from build123d import *

# Parameters (mm, degrees)
F0_W          = 23
F0_H          = 17.5
F1_DEPTH      = 10
F2_T          = -1.2
F3_R          = 5.7
F4_DEPTH      = 3
F3_R_2        = 6.7
F5_DEPTH      = 7.5
F6_W          = 6
F6_H          = 2.3
F6_W_2        = 3.5
F6_H_2        = 3.5
F7_DEPTH      = 4
F8_DEPTH      = 3
F10_DEPTH     = 30
F11_T1_DEPTH  = 19
F11_T3_DEPTH  = 23.5
F11_T5_DEPTH  = 13
F11_T7_DEPTH  = 27.8205080757
F11_S11_W     = 2
F11_S11_H     = 2
F11_T12_DEPTH = 2
F11_S17_W     = 2
F11_S17_H     = 2
F11_T18_DEPTH = 2


# Not quite as in the source:
# - a fillet or chamfer that OpenCascade refuses, or shapes differently, is made with other operations: its cross-section is extruded or revolved along the edge and cut away or added


with BuildPart() as f1:
    # F0 (on Front) → F1 (new body)
    with BuildSketch(Plane.XZ):
        Rectangle(F0_W, F0_H)
    extrude(amount=F1_DEPTH)

    # F2
    f2_openings = [f1.faces().sort_by_distance(p)[0] for p in [
        (0, -10, 0),
    ]]
    offset(amount=F2_T, openings=f2_openings)

    # F3 (on face) → F4 (cut)
    with BuildSketch(Plane(origin=(0, 0, 0), x_dir=(-1, 0, 0), z_dir=(0, 1, 0))):
        Circle(F3_R)
    extrude(amount=-F4_DEPTH, mode=Mode.SUBTRACT)

    # F3 (on face) → F5 (join)
    with BuildSketch(Plane(origin=(0, 0, 0), x_dir=(-1, 0, 0), z_dir=(0, 1, 0))):
        Circle(F3_R_2)
        Circle(F3_R, mode=Mode.SUBTRACT)
    extrude(amount=F5_DEPTH)

    # F6 (on face) → F7 (cut)
    with BuildSketch(Plane.XY.offset(8.75)):
        with Locations((1.5, -8.85)):
            Rectangle(F6_W, F6_H)
        with Locations((-5.75, -8.25)):
            Rectangle(F6_W_2, F6_H_2)
    extrude(amount=-F7_DEPTH, mode=Mode.SUBTRACT)

    # F8 (add): a face of the model
    f8_faces = [f1.faces().sort_by_distance(p)[0] for p in [
        (0, -5, -8.75),
    ]]
    extrude(f8_faces, amount=F8_DEPTH)

    # F9 (on face) → F10 (cut)
    with BuildSketch(Plane.YZ.offset(11.5)):
        Polygon((-10, -11.75), (0, -11.75), (-10, -9.0705080757), align=None)
    extrude(amount=-F10_DEPTH, mode=Mode.SUBTRACT)

    # F11: fillet of radius 2 on 7 edges, made by hand

    # F11_s2 → F11_t1 (cut)
    with BuildSketch(Plane.YZ.offset(-9.5)):
        with BuildLine():
            ThreePointArc((0, 6.75), (-0.5857864376, 8.1642135624), (-2, 8.75))
            Line((-2, 8.75), (0, 8.75))
            Line((0, 8.75), (0, 6.75))
        make_face()
    extrude(amount=F11_T1_DEPTH, mode=Mode.SUBTRACT)

    # F11_s4 → F11_t3 (cut)
    with BuildSketch(Plane.XY.offset(-16.75)):
        with BuildLine():
            ThreePointArc((-11.5, -2), (-10.9142135624, -0.5857864376), (-9.5, 0))
            Line((-9.5, 0), (-11.5, 0))
            Line((-11.5, 0), (-11.5, -2))
        make_face()
        with BuildLine():
            ThreePointArc((9.5, 0), (10.9142135624, -0.5857864376), (11.5, -2))
            Line((11.5, -2), (11.5, 0))
            Line((11.5, 0), (9.5, 0))
        make_face()
    extrude(amount=F11_T3_DEPTH, mode=Mode.SUBTRACT)

    # F11_s6 → F11_t5 (cut)
    with BuildSketch(Plane.XZ.offset(2)):
        with BuildLine():
            ThreePointArc((9.5, 8.75), (10.9142135624, 8.1642135624), (11.5, 6.75))
            Line((11.5, 6.75), (11.5, 8.75))
            Line((11.5, 8.75), (9.5, 8.75))
        make_face()
        with BuildLine():
            ThreePointArc((-11.5, 6.75), (-10.9142135624, 8.1642135624), (-9.5, 8.75))
            Line((-9.5, 8.75), (-11.5, 8.75))
            Line((-11.5, 8.75), (-11.5, 6.75))
        make_face()
    extrude(amount=F11_T5_DEPTH, mode=Mode.SUBTRACT)

    # F11_s8 → F11_t7 (cut)
    with BuildSketch(Plane.XY.offset(-14.0705080757)):
        with BuildLine():
            ThreePointArc((-11.5, -8), (-10.9142135624, -9.4142135624), (-9.5, -10))
            Line((-9.5, -10), (-11.5, -10))
            Line((-11.5, -10), (-11.5, -8))
        make_face()
        with BuildLine():
            ThreePointArc((9.5, -10), (10.9142135624, -9.4142135624), (11.5, -8))
            Line((11.5, -8), (11.5, -10))
            Line((11.5, -10), (9.5, -10))
        make_face()
    extrude(amount=F11_T7_DEPTH, mode=Mode.SUBTRACT)


with BuildPart() as f11_tool10:
    # F11_s11 → F11_t12 (new body)
    with BuildSketch(Plane.XZ.offset(2)):
        with Locations((10.5, 7.75)):
            Rectangle(F11_S11_W, F11_S11_H)
    extrude(amount=-F11_T12_DEPTH)

    # F11_s13 → F11_t14 (revolve, cut)
    with BuildSketch(Plane(origin=(9.5, -2, 6.75), x_dir=(-0.7071067812, 0, -0.7071067812), z_dir=(0.7071067812, 0, -0.7071067812))):
        with BuildLine():
            ThreePointArc((0, -2), (2, 0), (0, 2))
            Line((0, 2), (0, -2))
        make_face()
    revolve(axis=Axis((9.5, -2, 6.75), (0, 1, 0)), mode=Mode.SUBTRACT)


with BuildPart() as f1_1:
    add(f1.part)

    # F11_t9: cut F11_tool10
    add(f11_tool10.part, mode=Mode.SUBTRACT)


with BuildPart() as f11_tool16:
    # F11_s17 → F11_t18 (new body)
    with BuildSketch(Plane.YZ.offset(-9.5)):
        with Locations((-1, 7.75)):
            Rectangle(F11_S17_W, F11_S17_H)
    extrude(amount=-F11_T18_DEPTH)

    # F11_s19 → F11_t20 (revolve, cut)
    with BuildSketch(Plane(origin=(-9.5, -2, 6.75), x_dir=(0, -0.7071067812, -0.7071067812), z_dir=(0, 0.7071067812, -0.7071067812))):
        with BuildLine():
            ThreePointArc((0, -2), (2, 0), (0, 2))
            Line((0, 2), (0, -2))
        make_face()
    revolve(axis=Axis((-9.5, -2, 6.75), (-1, 0, 0)), mode=Mode.SUBTRACT)


with BuildPart() as f1_2:
    add(f1_1.part)

    # F11_t15: cut F11_tool16
    add(f11_tool16.part, mode=Mode.SUBTRACT)


solid = f1_2.part
Read the model definition and answer for the solid it produces. Units are mm, in the model's axes. A direction names the side the tool comes from. Give positions to 0.01 mm unless a question says otherwise; leave off trailing zeros. Write each loop counter-clockwise with the first axis right and the second up, starting at its lowest first coordinate (ties: lowest second). Pieces come first, ordered by that corner, then holes. Notation, with made-up numbers: (42, 52) -> (93, 52) arc R22 ccw to (93, 86) -> close; hole circle Ø4 at (18.25, 11). An arc over 180 degrees is marked (long way). Answer as a JSON object with one key per item and string values. Group by question number.
1) Find section C-C (y = 4.25). Write down the section's boundary in (x, z), and give its area (3 significant figures).
2) Find section A-A (x = 0). Write down the section's boundary in (y, z).
3) Each of these flat-tipped pins is pushed along its axis until it touches: P1, Ø5, axis at y = 3, z = -5.5, coming from the +X side; P2, Ø2, axis at x = -9, z = 1.5, coming from the -Y side; P3, Ø6, axis at x = 2, y = 2.5, coming from the +Z side. Where does it stop, or does it pass through?
4) Consider L1, parallel to X at y = -4.25, z = -6.5; L2, parallel to Y at x = -8.75, z = -1.25; L3, parallel to X at y = -8.75, z = -6. Determine where each line is inside the solid, lowest interval first. Write a range as from..to.
5) The mould has two halves that part along X. Classify faces 4 (the flat face through (-7.5, -8, 8)), 5 (the flat face through (0, -10, -8)), 6 (the flat face through (-4, -8, 8)), 7 (the cylindrical face through (-11.15, -9.13, -0.56)): +X half, -X half, draft (parallel to the pull), parting line (faces both ways), or undercut.
6) Find section D-D (z = -6). Write down the section's boundary in (x, y), and give its area (3 significant figures).
7) A tool of negligible diameter and unlimited length cuts with its end or side. For faces 1 (the flat face through (0, -5, 8.75)), 2 (the flat face through (-4.7, -1.2, 3.5)), 3 (the flat face through (-2.2, 0, -6.5)), from which of +Z, -Z, +X, -X, +Y, -Y can it reach the whole face along a straight path? Write none if from no direction.
8) Find section B-B (z = 0). Write down the section's boundary in (x, y).
Values follow:
{
 "1": {"outline": "circle Ø13.4 at (0, 0); hole circle Ø11.4 at (0, 0)", "area": "39.0 mm2"},
 "2": {"outline": "(-10, -9.07) -> (0, -11.75) -> (0, -6.7) -> (7.5, -6.7) -> (7.5, -5.7) -> (-1.2, -5.7) -> (-1.2, -7.55) -> (-10, -7.55) -> close; (-7.7, 7.55) -> (-1.2, 7.55) -> (-1.2, 5.7) -> (7.5, 5.7) -> (7.5, 6.7) -> (0, 6.7) -> (0, 6.75) arc R2 ccw to (-2, 8.75) -> (-7.7, 8.75) -> close"},
 "3": {"P1": "stops at x = 5.99", "P2": "stops at y = -1.2", "P3": "stops at z = 8.07"},
 "4": {"L1": "x = -11.5..-10.3, 10.3..11.5", "L2": "y = -1.2..0", "L3": "x = -11.35..-10.3, 10.3..11.35"},
 "5": {"face 4": "undercut", "face 5": "draft", "face 6": "undercut", "face 7": "-X half"},
 "6": {"outline": "(-11.5, -8) arc R2 ccw to (-10.3, -9.83) -> (-10.3, -1.2) -> (10.3, -1.2) -> (10.3, -9.83) arc R2 ccw to (11.5, -8) -> (11.5, -2) arc R2 ccw to (9.5, 0) -> (2.98, 0) -> (2.98, 7.5) -> (-2.98, 7.5) -> (-2.98, 0) -> (-9.5, 0) arc R2 ccw to (-11.5, -2) -> close", "area": "90.1 mm2"},
 "7": {"face 1": "+Z, +X, -X, +Y, -Y", "face 2": "-Y", "face 3": "+Y"},
 "8": {"outline": "(-11.5, -8) arc R2 ccw to (-10.3, -9.83) -> (-10.3, -1.2) -> (-5.7, -1.2) -> (-5.7, 7.5) -> (-6.7, 7.5) -> (-6.7, 0) -> (-9.5, 0) arc R2 ccw to (-11.5, -2) -> close; (5.7, -1.2) -> (10.3, -1.2) -> (10.3, -9.83) arc R2 ccw to (11.5, -8) -> (11.5, -2) arc R2 ccw to (9.5, 0) -> (6.7, 0) -> (6.7, 7.5) -> (5.7, 7.5) -> close"}
}
